Build history of the part. All positions in model axes, mm. Face numbers are marked on the shaded views. A direction names the side the tool comes from. Give positions to 0.01 mm unless a question says otherwise; leave off trailing zeros. Order: outer loops, then holes, each group sorted by start corner. A loop starts at its lowest first (then second) coordinate and runs counter-clockwise, first axis right, second up. Notation, with made-up numbers: M -10,-12.75 L 13,-12.75 A15 ccw 13,9.25 Z; hole C 75,-29.5 d7. An arc over 180 degrees is marked long. Answer as CSV lines item,"result".
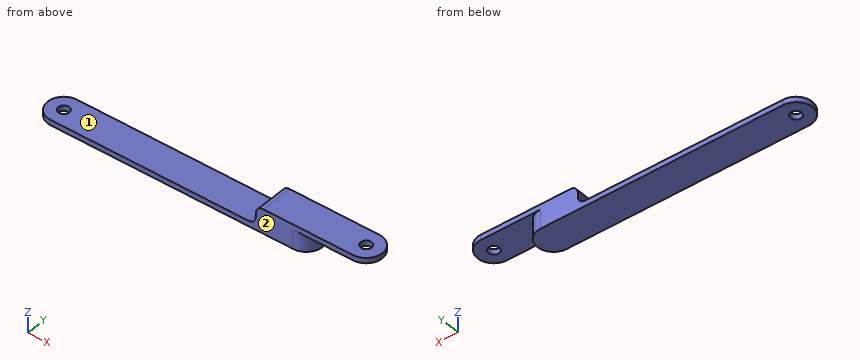
from build123d import *

# Parameters (mm, degrees)
BOSS_EXTRUDE1_DEPTH = 45
SKETCH2_R           = 5
CUT_EXTRUDE1_DEPTH  = 90
SKETCH7_OUTSIDE_W   = 279.254
SKETCH7_OUTSIDE_H   = 94.254
CUT_EXTRUDE2_DEPTH  = 50
FILLET1_R           = 7
BOSS_EXTRUDE2_DEPTH = 22.5
CUT_EXTRUDE3_START  = -17.6
SKETCH10_R          = 15
CUT_EXTRUDE3_DEPTH  = 17.6
FILLET3_START       = -1
FILLET3_DEPTH       = 18.6
CUT_EXTRUDE4_DEPTH  = 17.6
SKETCH12_R          = 5
CUT_EXTRUDE5_DEPTH  = 15


with BuildPart() as part:
    # Sketch1 → Boss-Extrude1 (new body)
    with BuildSketch(Plane.XY):
        with BuildLine():
            Line((0, 15), (200, 15))
            ThreePointArc((200, 15), (215, 0), (200, -15))
            Line((200, -15), (0, -15))
            ThreePointArc((0, -15), (-15, 0), (0, 15))
        make_face()
    extrude(amount=BOSS_EXTRUDE1_DEPTH)

    # Sketch2 → Cut-Extrude1 (cut)
    with BuildSketch(Plane.XY.offset(45)):
        Circle(SKETCH2_R)
    extrude(amount=-CUT_EXTRUDE1_DEPTH, mode=Mode.SUBTRACT)

    # Sketch7 outside → Cut-Extrude2 (cut)
    with BuildSketch(Plane.XZ.offset(15)):
        with Locations((100, 22.5)):
            Rectangle(SKETCH7_OUTSIDE_W, SKETCH7_OUTSIDE_H)
        Polygon((215, 22.5), (190, 22.5), (190, 5), (-15, 5), (-15, 0), (215, 0), align=None, mode=Mode.SUBTRACT)
    extrude(amount=-CUT_EXTRUDE2_DEPTH, mode=Mode.SUBTRACT)

    # Fillet1
    fillet1_edges = [part.edges().sort_by_distance(p)[0] for p in [
        (190, 0, 22.5),
        (190, 0, 5),
    ]]
    fillet(fillet1_edges, radius=FILLET1_R)

    # Sketch8 → Boss-Extrude2 (add)
    with BuildSketch(Plane.XY.offset(22.5)):
        with BuildLine():
            Line((200, 15), (280, 15))
            ThreePointArc((280, 15), (295, 0), (280, -15))
            Line((280, -15), (200, -15))
            Line((200, -15), (200, 15))
        make_face()
    extrude(amount=-BOSS_EXTRUDE2_DEPTH)

    # Sketch10 → Cut-Extrude3 (cut)
    with BuildSketch(Plane(origin=(0, 0, 0), x_dir=(-1, 0, 0), z_dir=(0, 0, -1)).offset(CUT_EXTRUDE3_START)):
        with Locations((-280, 0)):
            Circle(SKETCH10_R)
    extrude(amount=CUT_EXTRUDE3_DEPTH, mode=Mode.SUBTRACT)

    # Fillet3: read off the stored shape, not the designer's step
    # Fillet3 outline → Fillet3 (cut)
    with BuildSketch(Plane.XY.offset(FILLET3_START)):
        with BuildLine():
            ThreePointArc((280, -15), (271.538858878, -12.385842358), (266.026885319, -5.454545455))
            ThreePointArc((266.026885319, -5.454545455), (265.286158235, -11.948532524), (259.506098468, -15))
            Line((259.506098468, -15), (280, -15))
        make_face()
        with BuildLine():
            ThreePointArc((259.506098468, 15), (265.286158235, 11.948532524), (266.026885319, 5.454545455))
            ThreePointArc((266.026885319, 5.454545455), (271.538858878, 12.385842358), (280, 15))
            Line((280, 15), (259.506098468, 15))
        make_face()
    extrude(amount=FILLET3_DEPTH, mode=Mode.SUBTRACT)

    # Sketch11 → Cut-Extrude4 (cut)
    with BuildSketch(Plane(origin=(0, 0, 0), x_dir=(-1, 0, 0), z_dir=(0, 0, -1))):
        with BuildLine():
            Line((-224.645366828, -15), (-269.753049234, -15))
            Line((-269.753049234, -15), (-269.753049234, 15))
            Line((-269.753049234, 15), (-224.645366828, 15))
            ThreePointArc((-224.645366828, 15), (-239.645366828, 0), (-224.645366828, -15))
        make_face()
    extrude(amount=-CUT_EXTRUDE4_DEPTH, mode=Mode.SUBTRACT)

    # Sketch12 → Cut-Extrude5 (cut)
    with BuildSketch(Plane(origin=(0, 0, 17.6), x_dir=(-1, 0, 0), z_dir=(0, 0, -1))):
        with Locations((-280, 0)):
            Circle(SKETCH12_R)
    extrude(amount=-CUT_EXTRUDE5_DEPTH, mode=Mode.SUBTRACT)


solid = part.part
Item 1: Band-saw the part on B-B (x = 230). Give the cut face in (y, z).
Geometry says:
outline,"M -15,17.6 L -14.01,17.6 L -14.01,0 L 14.01,0 L 14.01,17.6 L 15,17.6 L 15,22.5 L -15,22.5 Z"
Item 2: Drop flat-ended pins along their axis: pin 1 (4 mm diameter, centred on y = 2, z = 10.5, fed in from +X); pin 2 (1 mm diameter, centred on y = 11, z = 10, fed in from +X); pin 3 (12 mm diameter, centred on x = 262, z = 16.5, fed in from +Y); pin 4 (6 mm diameter, centred on y = -12, z = 12.5, fed in from -X). Give the stop position or say it passes through.
Geometry says:
pin 1,"stops at x = 239.65"
pin 2,"stops at x = 235.36"
pin 3,"stops at y = 15"
pin 4,"stops at x = 189.54"
Item 3: Band-saw the part on C-C (x = 159.5). Give the cut face in (y, z), and give its area (3 significant figures).
Geometry says:
outline,"M -15,0 L 15,0 L 15,5 L -15,5 Z"
area,"150 mm2"
Item 4: Probe line 1 along Y through (x, z) = (280, 19.6); line 2 along Z through (x, y) = (82, 11); line 3 along X through (y, z) = (2.5, 20). List the from-to ranges inside material, lowest first. Write a range as from..to.
Geometry says:
line 1,"y = -15..-5, 5..15"
line 2,"z = 0..5"
line 3,"x = 191.64..275.67, 284.33..294.79"
Item 5: 3-axis set-ups, long thin cutter, end or side, ignore diameter. For the marked faces 1 and 2: which of +Z, -Z, +X, -X, +Y, -Y reach the whole face in a straight line?
Geometry says:
face 1,"+Z, -X, +Y, -Y"
face 2,"+Z, -Z, +X, -X, -Y"
Item 6: Band-saw the part on A-A (y = 0). Give the cut face in (x, z).
Geometry says:
outline,"M -15,0 L -5,0 L -5,5 L -15,5 Z; M 5,0 L 239.65,0 L 239.65,17.6 L 275,17.6 L 275,22.5 L 197,22.5 A7 ccw 190,15.5 L 190,12 A7 cw 183,5 L 5,5 Z; M 285,17.6 L 295,17.6 L 295,22.5 L 285,22.5 Z"
